Could you check a few things on this model? Use its own coordinates, in mm. A direction names the side the tool comes from. Round coordinates to 2 decimals unless told otherwise and drop trailing zeros. Write each loop counter-clockwise with the first axis right and the second up, starting at its lowest first coordinate (ties: lowest second). Pieces come first, ordered by that corner, then holes. Notation, with made-up numbers: (33.25, -16) -> (43.25, -16) arc R15 cw to (43.25, -7) -> close; hole circle Ø3 at (35.25, 21.25). An arc over 180 degrees is marked (long way). Answer in a Markdown table with one row per item. Add a question column.
```python
from build123d import *

# Parameters (mm, degrees)
SKETCH2_R                = 13.15
SKETCH2_R_2              = 8.15
BOSS_EXTRUDE1_DEPTH      = 25
BOSS_EXTRUDE2_DEPTH      = 13.15
BOSS_EXTRUDE2_DEPTH_BACK = 13.15
SKETCH4_R                = 8.15
CUT_EXTRUDE1_DEPTH       = 25
CUT_EXTRUDE2_START       = -25
SKETCH5_R                = 8.15
CUT_EXTRUDE2_DEPTH       = 25
FILLET1_R                = 10


with BuildPart() as part:
    # Sketch2 → Boss-Extrude1 (new body)
    # profile 1 of 5: a face of its own
    with BuildSketch(Plane(origin=(0, 0, 0), x_dir=(1, 0, 0), z_dir=(0, 1, 0))):
        with BuildLine():
            Line((-13.15, 13.15), (-13.15, 0))
            ThreePointArc((-13.15, 0), (-9.298454179, 9.298454166), (-1.9e-08, 13.15))
            Line((-1.9e-08, 13.15), (-13.15, 13.15))
        make_face()
    # profile 2 of 5: a face of its own
    with BuildSketch(Plane(origin=(0, 0, 0), x_dir=(1, 0, 0), z_dir=(0, 1, 0))):
        Circle(SKETCH2_R)
        with Locations(Location((0, 0, 0), (0, 0, 270))):
            Circle(SKETCH2_R_2, mode=Mode.SUBTRACT)
    # profile 3 of 5: a face of its own
    with BuildSketch(Plane(origin=(0, 0, 0), x_dir=(1, 0, 0), z_dir=(0, 1, 0))):
        with BuildLine():
            ThreePointArc((-1.9e-08, 13.15), (9.298454166, 9.298454179), (13.15, 0))
            Line((13.15, 0), (13.15, 13.15))
            Line((13.15, 13.15), (-1.9e-08, 13.15))
        make_face()
    # profile 4 of 5: a face of its own
    with BuildSketch(Plane(origin=(0, 0, 0), x_dir=(1, 0, 0), z_dir=(0, 1, 0))):
        with BuildLine():
            ThreePointArc((13.15, 0), (9.298454189, -9.298454156), (4.6e-08, -13.15))
            Line((4.6e-08, -13.15), (13.15, -13.15))
            Line((13.15, -13.15), (13.15, 0))
        make_face()
    # profile 5 of 5: a face of its own
    with BuildSketch(Plane(origin=(0, 0, 0), x_dir=(1, 0, 0), z_dir=(0, 1, 0))):
        with BuildLine():
            Line((-13.15, 0), (-13.15, -13.15))
            Line((-13.15, -13.15), (4.6e-08, -13.15))
            ThreePointArc((4.6e-08, -13.15), (-9.298454156, -9.298454189), (-13.15, 0))
        make_face()
    extrude(amount=BOSS_EXTRUDE1_DEPTH)

    # Sketch3 → Boss-Extrude2 (add, two sides: drawn at the far end of the back side and taken through both)
    with BuildSketch(Plane.XY.offset(-BOSS_EXTRUDE2_DEPTH_BACK)):
        with BuildLine():
            Line((-28.225635095, 1.11176594), (-6.575, -11.38823406))
            ThreePointArc((-6.575, -11.38823406), (11.38823406, -6.575), (6.575, 11.38823406))
            Line((6.575, 11.38823406), (-15.075635095, 23.88823406))
            Line((-15.075635095, 23.88823406), (-28.225635095, 1.11176594))
        make_face()
    extrude(amount=BOSS_EXTRUDE2_DEPTH + BOSS_EXTRUDE2_DEPTH_BACK)

    # Sketch4 → Cut-Extrude1 (cut)
    with BuildSketch(Plane(origin=(-21.650635095, 12.5, 0), x_dir=(0, 0, 1), z_dir=(-0.8660254037844418, 0.49999999999999445, 0))):
        with Locations(Location((0, 0, 0), (0, 0, 270))):
            Circle(SKETCH4_R)
    extrude(amount=-CUT_EXTRUDE1_DEPTH, mode=Mode.SUBTRACT)

    # Sketch5 → Cut-Extrude2 (cut)
    with BuildSketch(Plane(origin=(0, 25, 0), x_dir=(1, 0, 0), z_dir=(0, 1, 0)).offset(CUT_EXTRUDE2_START)):
        with Locations(Location((0, 0, 0), (0, 0, 270))):
            Circle(SKETCH5_R)
    extrude(amount=CUT_EXTRUDE2_DEPTH, mode=Mode.SUBTRACT)

    # Fillet1
    # the kernel refuses this fillet: 10 mm, written as the material it adds along each edge
    with BuildSketch(Plane(origin=(-13.15, 22.77646812, 13.15), x_dir=(0, 1, 0), z_dir=(0, 0, -1))) as fillet1_piece_1:
        with BuildLine():
            CenterArc((10.274215146, -5.93182088), FILLET1_R, 143.616854507, 12.766290987)
            Line((1.11176594, -1.925635095), (0, 0))
            Line((0, 0), (2.22353188, 0))
        make_face()
    extrude(amount=26.3)


solid = part.part
```
(1) Suppose I cut it at D-D, the plane y = -9.5. Please give me the cut outline in (x, z).
(2) Suppose I cut it at A-A, the plane z = 0. Please give me the cut outline in (x, y) (3 decimals), then the cut area to 3 significant figures.
(3) For P1, Ø1.5, axis at x = 7.5, z = 3.5, coming from the -Y side; P2, Ø3, axis at y = -8.5, z = -8, coming from the -X side; P3, Ø1, axis at x = -19, z = -8, coming from the +Y side, each with a flat end and sliding along its axis, tell me the tip position at first contact or that it passes through.
(4) If we mould it in two halves opening along X, with no side actions, what happens to faces 3 (the face through (3, 0, 0)), 4 (the face through (-17.55, -5.05, -0.18)), 5 (the face through (-3, 6, -13.15)), 6 (the face through (13.15, 12, 0))? For each: pulls with the +X half, pulls with the -X half, needs draft (parallel to the pull), parting line crosses it, or undercut.
(5) Suppose I cut it at C-C, the plane z = -10. Please give me the cut outline in (x, y) (3 decimals), then the cut area to 3 significant figures.
(6) Suppose I cut it at B-B, the plane x = 2.5. Please give me the cut outline in (y, z), then the cut area to 3 significant figures.
(7) I need wall thicknesses on L1, parallel to Z at x = -14.5, y = 8; L2, parallel to X at y = 10, z = 0; L3, parallel to X at y = -0.5, z = 2.5. Which ranges of each line are inside material? Lowest first, please.
(8) On a 3-axis mill with a long thin cutter (end or side, diameter ignored), from which of +Z, -Z, +X, -X, +Y, -Y can I reach the whole of each face in a straight line? I mean faces 1 (the face through (-1.56, -2.7, 0.11)), 2 (the face through (-6, 25, -6)). Say none if no direction works.
Response:
| question | item | result |
|---|---|---|
| 1 | outline | (-9.85, -13.15) -> (9.09, -13.15) -> (9.09, 13.15) -> (-9.85, 13.15) -> close |
| 2 | outline | (-28.226, 1.112) -> (-6.575, -11.388) arc R13.15 ccw to (13.15, 0) -> (13.15, 25) -> (8.15, 25) -> (8.15, 0) -> (0, 0) -> (-4.075, -7.058) -> (-25.726, 5.442) -> close; (-17.576, 19.558) -> (-8.15, 14.116) -> (-8.15, 25) -> (-13.15, 25) arc R10 cw to (-15.076, 23.888) -> close |
| 2 | area | 499 mm² |
| 3 | P1 | y = -11.29 |
| 3 | P2 | x = -14.18 |
| 3 | P3 | y = 17.96 |
| 4 | face 3 | undercut |
| 4 | face 4 | pulls with the -X half |
| 4 | face 5 | needs draft |
| 4 | face 6 | pulls with the +X half |
| 5 | outline | (-28.226, 1.112) -> (-6.575, -11.388) arc R13.15 ccw to (13.15, 0) -> (13.15, 25) -> (-13.15, 25) arc R10 cw to (-15.076, 23.888) -> close |
| 5 | area | 1,200 mm² |
| 6 | outline | (-12.91, -13.15) -> (25, -13.15) -> (25, -7.76) -> (0, -7.76) -> (0, 7.76) -> (25, 7.76) -> (25, 13.15) -> (-12.91, 13.15) -> close |
| 6 | area | 609 mm² |
| 7 | L1 | -13.15 to -8.14, 8.14 to 13.15 |
| 7 | L2 | 8.15 to 13.15 |
| 7 | L3 | -25.43 to -14.65, -0.29 to 13.14 |
| 8 | face 1 | +Y |
| 8 | face 2 | +Z, -Z, +X, -X, +Y |
